from build123d import *

# Parameters (mm, degrees)
CROQUIS1_W              = 68
CROQUIS1_H              = 5.5
CROQUIS1_R              = 0.75
CROQUIS1_R_2            = 1
SALIENTE_EXTRUIR1_DEPTH = 3
REDONDEO1_R             = 2.25


with BuildPart() as part:
    # Croquis1 → Saliente-Extruir1 (new body)
    with BuildSketch(Plane(origin=(0, 0, 0), x_dir=(1, 0, 0), z_dir=(0, 1, 0))):
        with Locations((4.363095238, 10.94047619)):
            Rectangle(CROQUIS1_W, CROQUIS1_H)
        with Locations((36.048095238, 10.94047619)):
            Circle(CROQUIS1_R, mode=Mode.SUBTRACT)
        with Locations((-26.636904762, 10.94047619)):
            Circle(CROQUIS1_R_2, mode=Mode.SUBTRACT)
    extrude(amount=SALIENTE_EXTRUIR1_DEPTH)

    # Redondeo1
    redondeo1_edges = [part.edges().sort_by_distance(p)[0] for p in [
        (-29.636904762, 1.5, -13.69047619),
        (38.363095238, 1.5, -13.69047619),
        (38.363095238, 1.5, -8.19047619),
        (-29.636904762, 1.5, -8.19047619),
    ]]
    fillet(redondeo1_edges, radius=REDONDEO1_R)


solid = part.part
The listing builds one solid part. Answer for the finished solid, in the listing's coordinates (mm). Round coordinates to 2 decimals unless told otherwise and drop trailing zeros. Loops run counter-clockwise (first coordinate to the right, second up) from the corner with the lowest first, then second, coordinate; pieces in that order, holes last. Notation, with made-up numbers: M 66.25,37.25 L 111.25,37.25 A21 ccw 111.25,72.25 Z; hole C 38.5,18.5 d3. An arc over 180 degrees is marked long. Write each question's results on one line, items separated by ' | '. Start each with the question number.
1) Find section B-B on z = -8.8. Write down the section's boundary in (x, y), plus the area to 3 significant figures.
2) Find section A-A on y = 1.55. Write down the section's boundary in (x, z), plus the area to 3 significant figures.
3) Straight lines are drawn through the part: probe 1 along X at (y, z) = (0.5, -10.9); probe 2 along X at (y, z) = (0.6, -10.3); probe 3 along X at (y, z) = (1.3, -9.85). For each, find the intervals that lie inside material, in ascending order.
4) Determine the mould class of faces 1 (the cylindrical face through (-27.636, 1.479, -10.984)), 2 (the flat face through (4, 3, -11)), 3 (the cylindrical face through (37.686, 1.521, -8.832)) for opening direction X: pulls with the +X half, pulls with the -X half, needs draft (parallel to the pull), parting line crosses it, or undercut.
Final values:
1) outline: M -28.93,0 L 37.65,0 L 37.65,3 L -28.93,3 Z | area: 200 mm²
2) outline: M -29.64,-11.44 A2.25 ccw -27.39,-13.69 L 36.11,-13.69 A2.25 ccw 38.36,-11.44 L 38.36,-10.44 A2.25 ccw 36.11,-8.19 L -27.39,-8.19 A2.25 ccw -29.64,-10.44 Z; hole C -26.64,-10.94 d2; hole C 36.05,-10.94 d1.5 | area: 365 mm²
3) probe 1: -29.64 to -27.64, -25.64 to 35.3, 36.8 to 38.36 | probe 2: -29.63 to -27.4, -25.87 to 35.66, 36.44 to 38.36 | probe 3: -29.56 to 38.28
4) face 1: undercut | face 2: needs draft | face 3: pulls with the +X half
